For this review, use the dimensioned drawing (mm, ordinates from the lowest corner) and the shaded views. A direction names the side the tool comes from. Give positions to 0.01 mm unless a question says otherwise; leave off trailing zeros. Write each loop counter-clockwise with the first axis right and the second up, starting at its lowest first coordinate (ties: lowest second). Pieces come first, ordered by that corner, then holes. Notation, with made-up numbers: M -2,79 L 29,79 A10 ccw 29,84 Z; hole C 25.25,7 d8. An arc over 180 degrees is marked long. Answer in a Markdown table with one row per item.
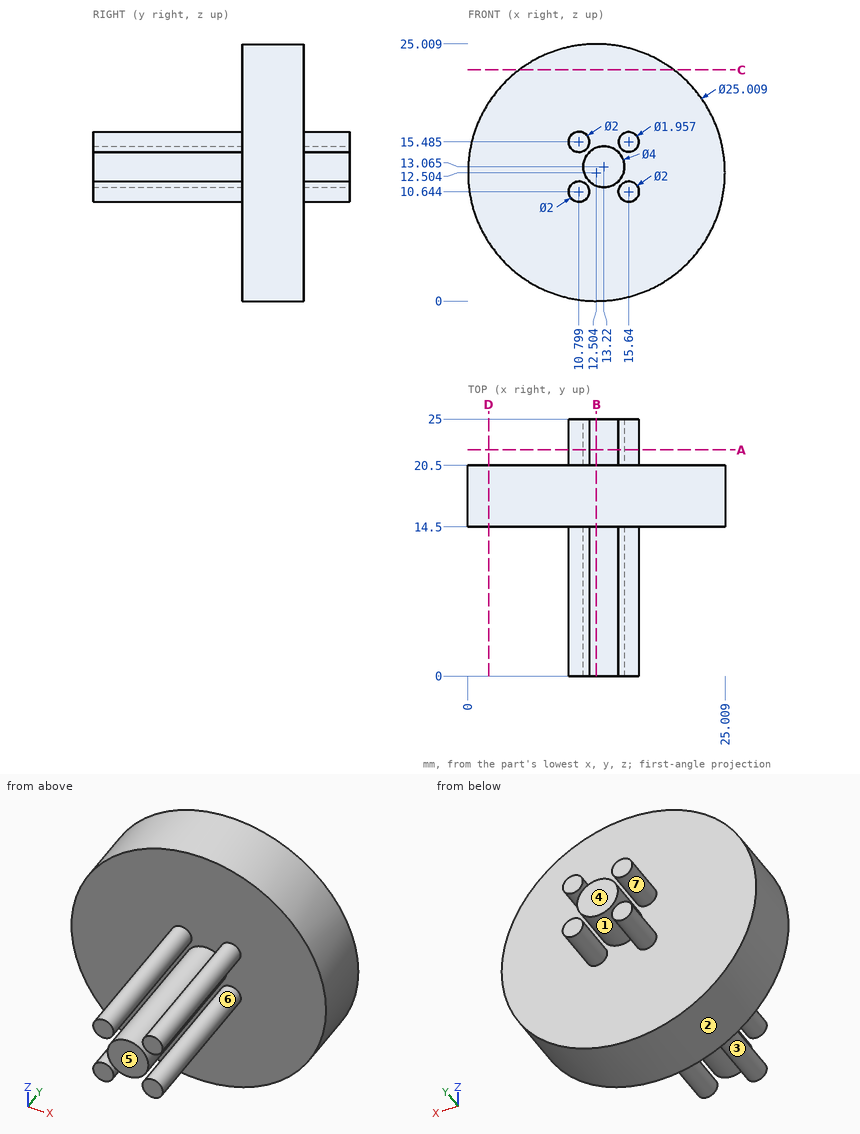
1) Insertion check: P1, Ø4, axis at x = 7, z = 22, coming from the +Y side; P2, Ø10, axis at y = 15, z = 7, coming from the -X side; P3, Ø6, axis at y = 11, z = 9.5, coming from the -X side. Each pin has a flat end and moves straight along its axis. Give the tip position at first contact, or say it passes through.
Geometry says:
| item | result |
|---|---|
| P1 | y = 20.5 |
| P2 | x = 0.01 |
| P3 | x = 9.8 |
2) Add section A-A (y = 22). Write out the cut boundary in (x, z) (1 decimal), and give its area (3 significant figures).
Geometry says:
| item | result |
|---|---|
| outline | C 10.8,10.6 d2; C 10.8,15.5 d2; C 13.2,13.1 d4; C 15.6,10.6 d2; C 15.6,15.5 d2 |
| area | 25.0 mm^2 |
3) To check wall thickness, follow probe 1 along Y at (x, z) = (9.5, 19.75); probe 2 along X at (y, z) = (22, 11.5) (1 decimal); probe 3 along Z at (x, y) = (10.5, 23.75). State the ranges of each line that lie inside material, in increasing order. Write a range as [from, to].
Geometry says:
| item | result |
|---|---|
| probe 1 | [14.5, 20.5] |
| probe 2 | [10.3, 11.3], [12, 14.5], [15.1, 16.2] |
| probe 3 | [9.69, 11.6], [14.53, 16.44] |
4) The part is to be moulded in two halves that separate along X. For the marked faces 1, 2, 3 and 4, say which applies: released by +X, released by -X, zero draft, split by the parting line, or undercut.
Geometry says:
| item | result |
|---|---|
| face 1 | undercut |
| face 2 | split by the parting line |
| face 3 | undercut |
| face 4 | zero draft |
5) Add section C-C (z = 22.5). Write out the cut boundary in (x, y).
Geometry says:
| item | result |
|---|---|
| outline | M 4.99,14.5 L 20.02,14.5 L 20.02,20.5 L 4.99,20.5 Z |
6) Add section B-B (x = 12.5). Write out the cut boundary in (y, z).
Geometry says:
| item | result |
|---|---|
| outline | M 0,11.2 L 14.5,11.2 L 14.5,0 L 20.5,0 L 20.5,11.2 L 25,11.2 L 25,14.93 L 20.5,14.93 L 20.5,25.01 L 14.5,25.01 L 14.5,14.93 L 0,14.93 Z |
7) For the marked faces 5, 6 and 7, list the 3-axis set-ups (+Z, -Z, +X, -X, +Y, -Y) from which the entire face can be reached by the end or side of a thin tool; tool diameter is ignored.
Geometry says:
| item | result |
|---|---|
| face 5 | +Z, -Z, +X, -X, -Y |
| face 6 | -Y |
| face 7 | +Y |
8) Add section D-D (x = 2). Write out the cut boundary in (y, z).
Geometry says:
| item | result |
|---|---|
| outline | M 14.5,5.72 L 20.5,5.72 L 20.5,19.29 L 14.5,19.29 Z |
